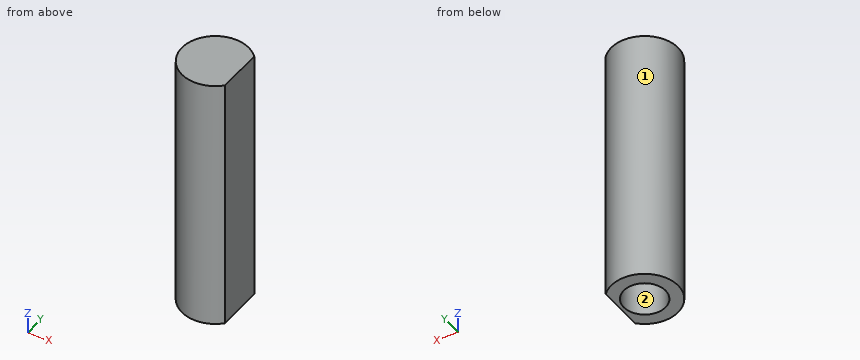
```python
from build123d import *

# Parameters (mm, degrees)
SALIENTE_EXTRUIR1_DEPTH = 31
SALIENTE_EXTRUIR2_START = -6.2
SALIENTE_EXTRUIR2_DEPTH = 6.2
CROQUIS5_R              = 2.5
CORTAR_EXTRUIR1_DEPTH   = 5


with BuildPart() as part:
    # Croquis1 → Saliente-Extruir1 (new body)
    with BuildSketch(Plane.XY):
        with BuildLine():
            Line((2.90473751, 2.75), (2.90473751, -2.75))
            ThreePointArc((2.90473751, -2.75), (-4, 0), (2.90473751, 2.75))
        make_face()
        with BuildLine():
            Line((2, 1.5), (2, -1.5))
            ThreePointArc((2, -1.5), (-2.5, 0), (2, 1.5))
        make_face(mode=Mode.SUBTRACT)
    extrude(amount=SALIENTE_EXTRUIR1_DEPTH)

    # Croquis2 → Saliente-Extruir2 (add)
    with BuildSketch(Plane.XY.offset(31).offset(SALIENTE_EXTRUIR2_START)):
        with BuildLine():
            Line((2.90473751, 2.75), (2.90473751, -2.75))
            ThreePointArc((2.90473751, -2.75), (-4, 0), (2.90473751, 2.75))
        make_face()
    extrude(amount=SALIENTE_EXTRUIR2_DEPTH)

    # Croquis5 → Cortar-Extruir1 (cut)
    with BuildSketch(Plane(origin=(0, 0, 0), x_dir=(-1, 0, 0), z_dir=(0, 0, -1))):
        with Locations(Location((0, 0, 0), (0, 0, 216.869897646))):
            Circle(CROQUIS5_R)
    extrude(amount=-CORTAR_EXTRUIR1_DEPTH, mode=Mode.SUBTRACT)


solid = part.part
```
CAD build for the part. Positions are in the model's coordinates, mm. Face numbers are marked on the shaded views. A direction names the side the tool comes from. Give positions to 0.01 mm unless a question says otherwise; leave off trailing zeros. Loops run counter-clockwise (first coordinate to the right, second up) from the corner with the lowest first, then second, coordinate; pieces in that order, holes last. Notation, with made-up numbers: (-25.75, 11.25) - (8.25, 11.25) arc R30 ccw to (8.25, 34.25) - close; hole circle Ø1 at (25, 24). An arc over 180 degrees is marked (long way). Put each result on its own line as item: value.
Q1. Probe line 1 along Y through (x, z) = (0, 14.5); line 2 along X through (y, z) = (0, 7.5); line 3 along Z through (x, y) = (-0.25, 0.75). List the from-to ranges inside material, lowest first.
Filled in:
line 1: y = -4 to -2.5, 2.5 to 4
line 2: x = -4 to -2.5, 2 to 2.9
line 3: z = 24.8 to 31
Q2. Tool access for the marked faces 1 and 2: list every direction of +Z, -Z, +X, -X, +Y, -Y with a clear straight run to the whole face (end or side of a thin tool).
Filled in:
face 1: +Z, -Z
face 2: -Z
Q3. Flat gauge pin, fed straight in: pin 1 (1.5 mm diameter, centred on x = 2, z = 28, fed in from -Y). Where does the tip first touch, or does it go through?
Filled in:
pin 1: stops at y = -3.8
Q4. Slice it at A-A (y = 0). Give the cut face in (x, z).
Filled in:
outline: (-4, 0) - (-2.5, 0) - (-2.5, 24.8) - (2, 24.8) - (2, 5) - (2.5, 5) - (2.5, 0) - (2.9, 0) - (2.9, 31) - (-4, 31) - close
Q5. Slice it at C-C (z = 13.5). Give the cut face in (x, y), plus the area to 3 significant figures.
Filled in:
outline: (2.9, -2.75) - (2.9, 2.75) arc R4 ccw (long way) to start; hole (2, -1.5) - (2, 1.5) arc R2.5 ccw (long way) to start
area: 27.5 mm²
Q6. Slice it at B-B (x = 0). Give the cut face in (y, z), plus the area to 3 significant figures.
Filled in:
outline: (-4, 0) - (-2.5, 0) - (-2.5, 24.8) - (2.5, 24.8) - (2.5, 0) - (4, 0) - (4, 31) - (-4, 31) - close
area: 124 mm²
